Input: part model. Units: mm. Frame: model coordinates. A direction names the side the tool comes from. Give positions to 0.01 mm unless a question says otherwise; leave off trailing zeros. Loops run counter-clockwise (first coordinate to the right, second up) from the corner with the lowest first, then second, coordinate; pieces in that order, holes last. Notation, with made-up numbers: (-16, 2) -> (39, 2) arc R30 cw to (39, 40) -> close; hole circle Ø3 at (41, 39). An arc over 180 degrees is marked (long way). Answer in a Markdown table with one row per item. Add a question column.
```python
from build123d import *

# Parameters (mm, degrees)
SKETCH1_R           = 2.7
SKETCH1_R_2         = 1.5
BOSS_EXTRUDE1_DEPTH = 5
SKETCH2_W           = 4.5
SKETCH2_H           = 5.9
BOSS_EXTRUDE2_DEPTH = 0.75
BOSS_EXTRUDE2_TAPER = 5


with BuildPart() as part:
    # Sketch1 → Boss-Extrude1 (new body)
    with BuildSketch(Plane.XY):
        with BuildLine():
            Line((0, -2), (0, -33))
            ThreePointArc((0, -33), (0.585786438, -34.414213562), (2, -35))
            Line((2, -35), (8.5, -35))
            ThreePointArc((8.5, -35), (9.914213562, -34.414213562), (10.5, -33))
            Line((10.5, -33), (10.5, -18))
            ThreePointArc((10.5, -18), (11.085786438, -16.585786438), (12.5, -16))
            Line((12.5, -16), (13, -16))
            ThreePointArc((13, -16), (14.414213562, -15.414213562), (15, -14))
            Line((15, -14), (15, -2))
            ThreePointArc((15, -2), (14.414213562, -0.585786438), (13, 0))
            Line((13, 0), (2, 0))
            ThreePointArc((2, 0), (0.585786438, -0.585786438), (0, -2))
        make_face()
        with Locations((7.5, -10)):
            Circle(SKETCH1_R, mode=Mode.SUBTRACT)
        with Locations((3, -29.8)):
            Circle(SKETCH1_R_2, mode=Mode.SUBTRACT)
        with Locations((3, -20.3)):
            Circle(SKETCH1_R_2, mode=Mode.SUBTRACT)
    extrude(amount=BOSS_EXTRUDE1_DEPTH)

    # Sketch2 → Boss-Extrude2 (add)
    with BuildSketch(Plane.XY.offset(5)):
        with Locations((2.25, -10)):
            Rectangle(SKETCH2_W, SKETCH2_H)
        with Locations((12.75, -10)):
            Rectangle(SKETCH2_W, SKETCH2_H)
    extrude(amount=BOSS_EXTRUDE2_DEPTH, taper=BOSS_EXTRUDE2_TAPER)


solid = part.part
```
1) Section D-D on x = 3. Output: boundary loops of the cut face in (y, z).
2) Pin query (flat end, axial travel): pin 1 (1.8 mm diameter, centred on x = 3, y = -29.8, fed in from +Z); pin 2 (5 mm diameter, centred on x = 8.5, y = -21.5, fed in from +Z); pin 3 (2.5 mm diameter, centred on y = -25.5, z = 2, fed in from +X). Return the tip coordinate at first contact, or that it passes through.
3) Reachability of faces 1 (the face through (10.5, -26, 2)), 2 (the face through (0.6, -0.57, 2.46)) from +Z, -Z, +X, -X, +Y, -Y: full face, straight path, thin tool, end or side. Return the list, or none.
4) Material intervals for line 1 along Y through (x, z) = (3, 1.75); line 2 along Y through (x, z) = (7.5, 1.25); line 3 along Z through (x, y) = (3.5, -25), sorted ascending.
5) Section A-A on y = -10. Output: boundary loops of the cut face in (x, z), and give its area (3 significant figures).
6) Pull-direction query (Y, two-part tool) for faces 3 (the face through (2.675, -31.264, 2.465)), 4 (the face through (11.07, -16.6, 2.46)), 5 (the face through (0, -17, 2)); classes: +Y half, -Y half, draft (parallel to the pull), parting line (faces both ways), or undercut.
7) Section B-B on x = 7.5. Output: boundary loops of the cut face in (y, z), and give its area (3 significant figures).
8) Section C-C on z = 1.2. Output: boundary loops of the cut face in (x, y).
Working result:
| question | item | result |
|---|---|---|
| 1 | outline | (-35, 0) -> (-31.3, 0) -> (-31.3, 5) -> (-35, 5) -> close; (-28.3, 0) -> (-21.8, 0) -> (-21.8, 5) -> (-28.3, 5) -> close; (-18.8, 0) -> (0, 0) -> (0, 5) -> (-7.05, 5) -> (-7.12, 5.75) -> (-12.88, 5.75) -> (-12.95, 5) -> (-18.8, 5) -> close |
| 2 | pin 1 | passes through |
| 2 | pin 2 | stops at z = 5 |
| 2 | pin 3 | stops at x = 10.5 |
| 3 | face 1 | +Z, -Z, +X, -Y |
| 3 | face 2 | +Z, -Z, -X, +Y |
| 4 | line 1 | y = -35 to -31.3, -28.3 to -21.8, -18.8 to 0 |
| 4 | line 2 | y = -35 to -12.7, -7.3 to 0 |
| 4 | line 3 | z = 0 to 5 |
| 5 | outline | (0, 0) -> (4.8, 0) -> (4.8, 5) -> (4.5, 5) -> (4.43, 5.75) -> (0.07, 5.75) -> (0, 5) -> close; (10.2, 0) -> (15, 0) -> (15, 5) -> (14.93, 5.75) -> (10.57, 5.75) -> (10.5, 5) -> (10.2, 5) -> close |
| 5 | area | 54.7 mm2 |
| 6 | face 3 | undercut |
| 6 | face 4 | -Y half |
| 6 | face 5 | draft |
| 7 | outline | (-35, 0) -> (-12.7, 0) -> (-12.7, 5) -> (-35, 5) -> close; (-7.3, 0) -> (0, 0) -> (0, 5) -> (-7.3, 5) -> close |
| 7 | area | 148 mm2 |
| 8 | outline | (0, -33) arc R2 ccw to (2, -35) -> (8.5, -35) arc R2 ccw to (10.5, -33) -> (10.5, -18) arc R2 cw to (12.5, -16) -> (13, -16) arc R2 ccw to (15, -14) -> (15, -2) arc R2 ccw to (13, 0) -> (2, 0) arc R2 ccw to (0, -2) -> close; hole circle Ø3 at (3, -29.8); hole circle Ø3 at (3, -20.3); hole circle Ø5.4 at (7.5, -10) |
